```python
from build123d import *

# Parameters (mm, degrees)
SKETCH1_W                                           = 20
SKETCH1_H                                           = 55
BOSS_EXTRUDE1_DEPTH                                 = 20
SKETCH2_R                                           = 4
CUT_EXTRUDE1_DEPTH                                  = 10
SKETCH3_W                                           = 20
SKETCH3_H                                           = 20
CUT_EXTRUDE2_DEPTH                                  = 10
CBORE_FOR_M3_HEX_SOCKET_HEAD_CAP_SCREW1_D           = 3.4
CBORE_FOR_M3_HEX_SOCKET_HEAD_CAP_SCREW1_CBORE_D     = 6.5
CBORE_FOR_M3_HEX_SOCKET_HEAD_CAP_SCREW1_CBORE_DEPTH = 3.4
FILLET2_R                                           = 5
SKETCH9_R                                           = 2.25
CUT_EXTRUDE5_DEPTH                                  = 40.449334595
CUT_EXTRUDE6_DEPTH                                  = 4
FILLET5_R                                           = 3


with BuildPart() as part:
    # Sketch1 → Boss-Extrude1 (new body)
    with BuildSketch(Plane(origin=(0, 0, 0), x_dir=(1, 0, 0), z_dir=(0, 1, 0))):
        Rectangle(SKETCH1_W, SKETCH1_H)
    extrude(amount=BOSS_EXTRUDE1_DEPTH)

    # Sketch2 → Cut-Extrude1 (cut)
    with BuildSketch(Plane(origin=(0, 20, 0), x_dir=(1, 0, 0), z_dir=(0, 1, 0))):
        with Locations(Location((-3, 0, 0), (0, 0, 270))):
            Circle(SKETCH2_R)
    extrude(amount=-CUT_EXTRUDE1_DEPTH, mode=Mode.SUBTRACT)

    # Sketch3 → Cut-Extrude2 (cut)
    with BuildSketch(Plane(origin=(0, 20, 0), x_dir=(1, 0, 0), z_dir=(0, 1, 0))):
        with Locations((0, -17.5)):
            Rectangle(SKETCH3_W, SKETCH3_H)
        with Locations((0, 17.5)):
            Rectangle(SKETCH3_W, SKETCH3_H)
    extrude(amount=-CUT_EXTRUDE2_DEPTH, mode=Mode.SUBTRACT)

    # CBORE for M3 Hex Socket Head Cap Screw1 (through all)
    with Locations(Plane(origin=(0, 10, 0), x_dir=(1, 0, 0), z_dir=(0, 1, 0))):
        with Locations((0, -15.5), (0, 15.5)):
            CounterBoreHole(CBORE_FOR_M3_HEX_SOCKET_HEAD_CAP_SCREW1_D / 2, CBORE_FOR_M3_HEX_SOCKET_HEAD_CAP_SCREW1_CBORE_D / 2, CBORE_FOR_M3_HEX_SOCKET_HEAD_CAP_SCREW1_CBORE_DEPTH)

    # Fillet2
    fillet2_edges = [part.edges().sort_by_distance(p)[0] for p in [
        (-10, 15, 7.5),
        (10, 15, 7.5),
        (-10, 15, -7.5),
        (10, 15, -7.5),
    ]]
    fillet(fillet2_edges, radius=FILLET2_R)

    # Sketch9 → Cut-Extrude5 (cut, through all)
    with BuildSketch(Plane.ZY.offset(10)):
        with Locations((-21, 5)):
            Circle(SKETCH9_R)
        with Locations((21, 5)):
            Circle(SKETCH9_R)
    extrude(amount=-CUT_EXTRUDE5_DEPTH, mode=Mode.SUBTRACT)

    # Sketch10 → Cut-Extrude6 (cut)
    with BuildSketch(Plane(origin=(10, 0, 0), x_dir=(0, 0, -1), z_dir=(1, 0, 0))):
        Polygon((-16.958548116, 5), (-18.979274058, 8.5), (-23.020725942, 8.5), (-25.041451884, 5), (-23.020725942, 1.5), (-18.979274058, 1.5), align=None)
        Polygon((16.958548116, 5), (18.979274058, 1.5), (23.020725942, 1.5), (25.041451884, 5), (23.020725942, 8.5), (18.979274058, 8.5), align=None)
    extrude(amount=-CUT_EXTRUDE6_DEPTH, mode=Mode.SUBTRACT)

    # Fillet5
    fillet5_edges = [part.edges().sort_by_distance(p)[0] for p in [
        (0, 10, 27.5),
        (0, 10, -27.5),
    ]]
    fillet(fillet5_edges, radius=FILLET5_R)


solid = part.part
```
Part model, mm, in its own coordinate system. A direction names the side the tool comes from. Round coordinates to 2 decimals unless told otherwise and drop trailing zeros. Write each loop counter-clockwise with the first axis right and the second up, starting at its lowest first coordinate (ties: lowest second). Pieces come first, ordered by that corner, then holes. Notation, with made-up numbers: (35, 27.25) -> (85, 27.25) arc R30 ccw to (85, 66.25) -> close; hole circle Ø4 at (6.25, -31.75). An arc over 180 degrees is marked (long way). Return JSON: item names as keys, results as strings. Group by question number.
Q1. Mould opens along Y. For faces 6 (the flat face through (2, 20, 0)), 7 (the flat face through (0, 0, 0)), 8 (the flat face through (8, 6.8, 24)), 9 (the cylindrical face through (-0.423, 8.324, -18.722)) say: pulls with the +Y half, pulls with the -Y half, needs draft (parallel to the pull), parting line crosses it, or undercut.
Q2. Saw through at B-B on y = 4. Write the cut outline in (x, z).
Q3. Which spindle directions (+Z, -Z, +X, -X, +Y, -Y) get a long thin tool onto all of the face, cutting with end or side? Do faces 1 (the flat face through (6, 7, 19)), 2 (the cylindrical face through (-5.4, 15.1, -3.2)), 3 (the cylindrical face through (-8.57, 14.93, 6)), 4 (the flat face through (0, 15, -7.5)), 5 (the flat face through (0, 3, 27.5)). Say none if no direction does.
Q4. Saw through at C-C on y = 13. Write the cut outline in (x, z).
Q5. Pin check, flat tips, straight feed: pin 1 (3 mm diameter, centred on x = -1, y = 16.5, fed in from -Z); pin 2 (4.5 mm diameter, centred on x = 0, z = 15.5, fed in from +Y); pin 3 (5 mm diameter, centred on x = -1, y = 13, fed in from +Z). Stop position of each tip, or through.
Q6. Saw through at D-D on x = 2.75. Write the cut outline in (y, z), plus the area to 3 significant figures.
Q7. Saw through at A-A on z = 15.5. Write the cut outline in (x, y).
Q8. Probe L1, parallel to Z at x = -3.5, y = 6; L2, parallel to Y at x = 7.5, z = -20; L3, parallel to Z at x = 0, y = 3.75. List the from-to ranges inside material, lowest first. Write a range as [from, to].
Answer:
{
 "1": {"face 6": "pulls with the +Y half", "face 7": "pulls with the -Y half", "face 8": "undercut", "face 9": "needs draft"},
 "2": {"outline": "(-10, -27.5) -> (10, -27.5) -> (10, -24.46) -> (6, -24.46) -> (6, -23.02) -> (-10, -23.02) -> close; (-10, -18.98) -> (6, -18.98) -> (6, -17.54) -> (10, -17.54) -> (10, 17.54) -> (6, 17.54) -> (6, 18.98) -> (-10, 18.98) -> close; (-10, 23.02) -> (6, 23.02) -> (6, 24.46) -> (10, 24.46) -> (10, 27.5) -> (-10, 27.5) -> close; hole circle Ø3.4 at (0, -15.5); hole circle Ø3.4 at (0, 15.5)"},
 "3": {"face 1": "+X", "face 2": "+Y", "face 3": "+Z, -X, +Y", "face 4": "-Z, +X, -X, +Y", "face 5": "+Z, +X, -X, +Y, -Y"},
 "4": {"outline": "(-10, -2.5) arc R5 ccw to (-5, -7.5) -> (5, -7.5) arc R5 ccw to (10, -2.5) -> (10, 2.5) arc R5 ccw to (5, 7.5) -> (-5, 7.5) arc R5 ccw to (-10, 2.5) -> close; hole circle Ø8 at (-3, 0)"},
 "5": {"pin 1": "z = -7.5", "pin 2": "y = 6.6", "pin 3": "z = 7.5"},
 "6": {"outline": "(0, -27.5) -> (7, -27.5) arc R3 ccw to (10, -24.5) -> (10, -17.23) -> (6.6, -17.23) -> (6.6, -13.77) -> (10, -13.77) -> (10, -7.5) -> (20, -7.5) -> (20, 7.5) -> (10, 7.5) -> (10, 13.77) -> (6.6, 13.77) -> (6.6, 17.23) -> (10, 17.23) -> (10, 24.5) arc R3 ccw to (7, 27.5) -> (0, 27.5) -> close; hole circle Ø4.5 at (5, -21); hole circle Ø4.5 at (5, 21)", "area": "641 mm2"},
 "7": {"outline": "(-10, 0) -> (-1.7, 0) -> (-1.7, 6.6) -> (-3.25, 6.6) -> (-3.25, 10) -> (-10, 10) -> close; (1.7, 0) -> (10, 0) -> (10, 10) -> (3.25, 10) -> (3.25, 6.6) -> (1.7, 6.6) -> close"},
 "8": {"L1": "[-27.5, -23.02], [-18.98, 18.98], [23.02, 27.5]", "L2": "[0, 1.5], [8.5, 10]", "L3": "[-27.5, -22.87], [-19.13, -17.2], [-13.8, 13.8], [17.2, 19.13], [22.87, 27.5]"}
}
